```python
from build123d import *

# Parameters (mm, degrees)
SKETCH_1_W          = 3
SKETCH_1_H          = 70
SKETCH_1_W_2        = 90
EXTRUDE_1_DEPTH     = 3
SKETCH_1_3_W        = 3
SKETCH_1_3_H        = 70
EXTRUDE_2_DEPTH     = 34
SKETCH_2_W          = 20
SKETCH_2_H          = 3
EXTRUDE_3_DEPTH     = 8
SKETCH_3_R          = 1.5
CUT_EXTRUDE_1_DEPTH = 8
SKETCH_5_W          = 70
SKETCH_5_H          = 2
EXTRUDE_4_DEPTH     = 10
SKETCH_4_R          = 1.5
CUT_EXTRUDE_2_DEPTH = 2
SKETCH_6_W          = 7
SKETCH_6_H          = 28
CUT_EXTRUDE_3_DEPTH = 2
FILLET_1_R          = 3
SKETCH_7_W          = 14
SKETCH_7_H          = 14
SKETCH_7_W_2        = 7
CUT_EXTRUDE_4_DEPTH = 3
SKETCH_8_W          = 14
SKETCH_8_H          = 14
SKETCH_8_W_2        = 7
CUT_EXTRUDE_5_DEPTH = 3
SKETCH_9_W          = 70.71367567
SKETCH_9_H          = 40.396420294
CUT_EXTRUDE_6_DEPTH = 3
CUT_EXTRUDE_7_REACH = 116.878
SKETCH_10_W         = 27.669088334
SKETCH_10_H         = 18.732687127
CHAMFER_1_SIZE      = 2
CHAMFER_1_SIZE2     = 1.678199262


with BuildPart() as part:
    # 草图1 → 凸台-拉伸1 (new body)
    with BuildSketch(Plane(origin=(0, 0, 0), x_dir=(1, 0, 0), z_dir=(0, 1, 0))):
        with Locations((-46.5, 0)):
            Rectangle(SKETCH_1_W, SKETCH_1_H)
        Rectangle(SKETCH_1_W_2, SKETCH_1_H)
        with Locations((46.5, 0)):
            Rectangle(SKETCH_1_W, SKETCH_1_H)
    extrude(amount=EXTRUDE_1_DEPTH)

    # 草图1<3> → 凸台-拉伸2 (add)
    with BuildSketch(Plane(origin=(0, 0, 0), x_dir=(1, 0, 0), z_dir=(0, 1, 0))):
        with Locations((-46.5, 0)):
            Rectangle(SKETCH_1_3_W, SKETCH_1_3_H)
        with Locations((46.5, 0)):
            Rectangle(SKETCH_1_3_W, SKETCH_1_3_H)
    extrude(amount=-EXTRUDE_2_DEPTH)

    # 草图2 → 凸台-拉伸3 (add)
    with BuildSketch(Plane.ZY.offset(48)):
        with Locations((0, -32.5)):
            Rectangle(SKETCH_2_W, SKETCH_2_H)
    extrude_3 = extrude(amount=EXTRUDE_3_DEPTH)

    # 镜向1: 凸台-拉伸3 across plane
    add(extrude_3.mirror(Plane(origin=(0, 0, 0), x_dir=(0, 0, 1), z_dir=(1, 0, 0))))

    # 草图3 → 切除-拉伸1 (cut)
    with BuildSketch(Plane(origin=(0, -31, 0), x_dir=(1, 0, 0), z_dir=(0, 1, 0))):
        with Locations(Location((-52, 6, 0), (0, 0, 270))):
            Circle(SKETCH_3_R)
        with Locations(Location((-52, -6, 0), (0, 0, 270))):
            Circle(SKETCH_3_R)
    cut_extrude_1 = extrude(amount=-CUT_EXTRUDE_1_DEPTH, mode=Mode.SUBTRACT)

    # 镜向3: 切除-拉伸1 across plane
    add(cut_extrude_1.mirror(Plane(origin=(0, 0, 0), x_dir=(0, 0, 1), z_dir=(1, 0, 0))), mode=Mode.SUBTRACT)

    # 草图5 → 凸台-拉伸4 (add)
    with BuildSketch(Plane.ZY.offset(48)):
        with Locations((0, 2)):
            Rectangle(SKETCH_5_W, SKETCH_5_H)
    extrude(amount=EXTRUDE_4_DEPTH)

    # 草图4 → 切除-拉伸2 (cut)
    with BuildSketch(Plane(origin=(0, 3, 0), x_dir=(1, 0, 0), z_dir=(0, 1, 0))):
        with Locations(Location((-55, 25, 0), (0, 0, 270))):
            Circle(SKETCH_4_R)
        with Locations(Location((-55, -25, 0), (0, 0, 270))):
            Circle(SKETCH_4_R)
        with Locations(Location((2, 31, 0), (0, 0, 270))):
            Circle(SKETCH_4_R)
        with Locations(Location((2, -31, 0), (0, 0, 270))):
            Circle(SKETCH_4_R)
    extrude(amount=-CUT_EXTRUDE_2_DEPTH, mode=Mode.SUBTRACT)

    # 草图6 → 切除-拉伸3 (cut)
    with BuildSketch(Plane(origin=(0, 3, 0), x_dir=(1, 0, 0), z_dir=(0, 1, 0))):
        with Locations((-54.5, 0)):
            Rectangle(SKETCH_6_W, SKETCH_6_H)
    extrude(amount=-CUT_EXTRUDE_3_DEPTH, mode=Mode.SUBTRACT)

    # 圆角1
    fillet_1_edges = [part.edges().sort_by_distance(p)[0] for p in [
        (-58, 2, 14),
        (-58, 2, -14),
        (-51, 2, -14),
        (-51, 2, 14),
    ]]
    fillet(fillet_1_edges, radius=FILLET_1_R)

    # 草图7 → 切除-拉伸4 (cut)
    with BuildSketch(Plane.ZY.offset(-45)):
        with Locations((28, -27)):
            Rectangle(SKETCH_7_W, SKETCH_7_H)
        with Locations((-31.5, -27)):
            Rectangle(SKETCH_7_W_2, SKETCH_7_H)
    extrude(amount=-CUT_EXTRUDE_4_DEPTH, mode=Mode.SUBTRACT)

    # 草图8 → 切除-拉伸5 (cut)
    with BuildSketch(Plane.ZY.offset(48)):
        with Locations((28, -27)):
            Rectangle(SKETCH_8_W, SKETCH_8_H)
        with Locations((-31.5, -27)):
            Rectangle(SKETCH_8_W_2, SKETCH_8_H)
    extrude(amount=-CUT_EXTRUDE_5_DEPTH, mode=Mode.SUBTRACT)

    # 草图9 → 切除-拉伸6 (cut)
    with BuildSketch(Plane(origin=(0, 3, 0), x_dir=(1, 0, 0), z_dir=(0, 1, 0))):
        with Locations((-0.249939669, 0.491140899)):
            Rectangle(SKETCH_9_W, SKETCH_9_H)
    extrude(amount=-CUT_EXTRUDE_6_DEPTH, mode=Mode.SUBTRACT)

    # 切除-拉伸7: up to this face of the body (flat: up to its plane)
    cut_extrude_7_end = Plane(part.part.faces().sort_by_distance((48, -13.531753131, -1.073792487))[0])
    # 草图10 → 切除-拉伸7 (cut, up to the picked face)
    with BuildSketch(Plane.ZY.offset(48), mode=Mode.PRIVATE) as cut_extrude_7_sk1:
        with Locations((-3.501584346, -13.325871908)):
            Rectangle(SKETCH_10_W, SKETCH_10_H)
    cut_extrude_7_tool1 = split(extrude(cut_extrude_7_sk1.sketch, amount=-CUT_EXTRUDE_7_REACH, mode=Mode.PRIVATE), bisect_by=cut_extrude_7_end, keep=Keep.BOTH, mode=Mode.PRIVATE)
    add(cut_extrude_7_tool1.solids().sort_by(Axis((-48, -13.325872, -3.501584), (1, 0, 0)))[0], mode=Mode.SUBTRACT)

    # 倒角1
    chamfer_1_edges = [part.edges().sort_by_distance(p)[0] for p in [
        (-48, 1, 0),
    ]]
    chamfer_1_side = [part.faces().sort_by_distance(p)[0] for p in [
        (-48, -33.217376208, -19),
    ]]
    chamfer(chamfer_1_edges, length=CHAMFER_1_SIZE, length2=CHAMFER_1_SIZE2, reference=chamfer_1_side[0])


solid = part.part
```
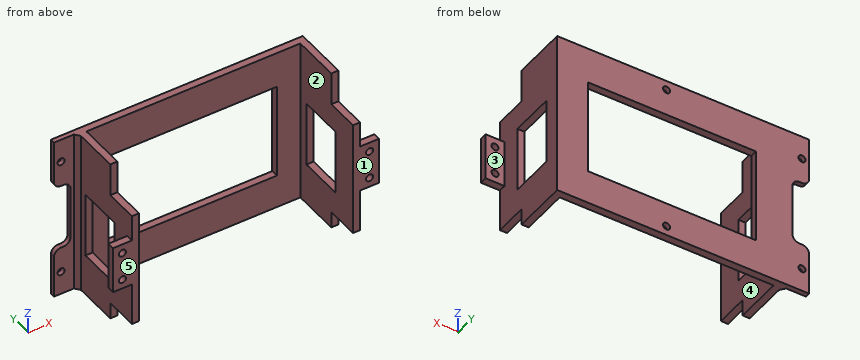
Here's how the part is built. I have some questions about the finished solid (model axes, mm). Face numbers are marked on the shaded views. A direction names the side the tool comes from. Give positions to 0.01 mm unless a question says otherwise; leave off trailing zeros. Write each loop counter-clockwise with the first axis right and the second up, starting at its lowest first coordinate (ties: lowest second). Pieces come first, ordered by that corner, then holes. Notation, with made-up numbers: M -32,2.25 L 26,2.25 A26 cw 26,37.25 Z; hole C 80.25,-9.75 d8. An arc over 180 degrees is marked long. Put each result on its own line as item: value. Start each with the question number.
Item 1: If we section it at D-D, the plane x = -32.5: Write out the boundary of the cut face in (y, z).
Item 2: If we section it at A-A, the plane x = 52: Write out the boundary of the cut face in (y, z), then the cut area to 3 significant figures.
Item 3: If we section it at B-B, the plane z = 25: Write out the boundary of the cut face in (x, y).
Item 4: If we section it at C-C, the plane y = -15: Write out the boundary of the cut face in (x, z), then the cut area to 3 significant figures.
Item 5: Thinking about a two-plate mould opening in X: for the marked faces 1 and 2, which applies, +X half, -X half, draft (parallel to the pull), parting line (faces both ways), or undercut?
Item 6: Will these pins go through, and if not, where does the flat tip stop? pin 1 (10 mm diameter, centred on x = 36, y = -7, fed in from +Z) (3 decimals); pin 2 (10 mm diameter, centred on y = -30, z = 24, fed in from +X); pin 3 (8 mm diameter, centred on x = -36, z = 5, fed in from -Y); pin 4 (0.9 mm diameter, centred on x = 46.5, y = -24, fed in from +Z).
Item 7: I need wall thicknesses on L1, parallel to Z at x = 52, y = -33.3; L2, parallel to X at y = -33.15, z = 6; L3, parallel to X at y = -18.5, z = 19. Which ranges of each line are inside material? Lowest first, please. Write a range as from..to.
Item 8: On a 3-axis mill with a long thin cutter (end or side, diameter ignored), from which of +Z, -Z, +X, -X, +Y, -Y can I reach the whole of each face in a straight line? I mean the marked faces 3, 4 and 5. Say none if no direction works.
Values:
1. outline: M 0,-35 L 3,-35 L 3,-20.69 L 0,-20.69 Z; M 0,19.71 L 3,19.71 L 3,35 L 0,35 Z
2. outline: M -34,-10 L -31,-10 L -31,-7.5 L -34,-7.5 Z; M -34,-4.5 L -31,-4.5 L -31,4.5 L -34,4.5 Z; M -34,7.5 L -31,7.5 L -31,10 L -34,10 Z
2. area: 42.0 mm²
3. outline: M -58,1 L -56.5,1 L -56.5,3 L -58,3 Z; M -53.5,1 L -49.68,1 L -48,-1 L -48,-20 L -45,-20 L -45,0 L 45,0 L 45,-20 L 48,-20 L 48,3 L -53.5,3 Z
4. outline: M -48,-35 L -45,-35 L -45,-17.34 L -48,-17.34 Z; M -48,10.33 L -45,10.33 L -45,35 L -48,35 Z; M 45,-35 L 48,-35 L 48,-17.34 L 45,-17.34 Z; M 45,10.33 L 48,10.33 L 48,35 L 45,35 Z
4. area: 254 mm²
5. face 1: draft
5. face 2: undercut
6. pin 1: through
6. pin 2: x = 48
6. pin 3: y = 0
6. pin 4: z = 21
7. L1: -10..-7.5, -4.5..4.5, 7.5..10
7. L2: -56..-53.5, -50.5..-45, 45..50.5, 53.5..56
7. L3: -48..-45, 45..48
8. face 3: +Z, -Z, +X, +Y
8. face 4: +Z, -Z, -Y
8. face 5: +Z, -Z, +X, -X, -Y
